Could you check a few things on this model? Use its own coordinates, in mm. Give positions to 0.01 mm unless a question says otherwise; leave off trailing zeros. Order: outer loops, then holes, each group sorted by start corner. A loop starts at its lowest first (then second) coordinate and runs counter-clockwise, first axis right, second up. Notation, with made-up numbers: (-12.5, 68) - (32.5, 68) arc R5 ccw to (32.5, 76) - close; hole circle Ø11 at (4, 82.5). An arc over 180 degrees is marked (long way). Put each result on its own line as item: value.
from build123d import *

# Parameters (mm, degrees)
F2_R     = 5.25
F4_R     = 25.9807621135
F5_DEPTH = 2.5


# Not quite as in the source:
# - a pattern or mirror of a feature is missing from the dataset's text; its kind, count and spacing are read off the source's solid


with BuildPart() as f1:
    # F0 (on Front) → F1 (revolve)
    with BuildSketch(Plane.XZ):
        with BuildLine():
            Line((-15, 25.9807621135), (-15, 0))
            Line((-15, 0), (15, 0))
            Line((15, 0), (15, 25.9807621135))
            ThreePointArc((15, 25.9807621135), (0, 30), (-15, 25.9807621135))
        make_face()
    revolve(axis=Axis((0, 0, 0), (1, 0, 0)))

    # F2 (on Right) → F3 (revolve, cut)
    with BuildSketch(Plane.YZ):
        with Locations((0, -27.5)):
            Circle(F2_R)
    f3 = revolve(axis=Axis((0, 15, 0), (0, 1, 0)), mode=Mode.SUBTRACT)

    # F3_copies: F3 across plane
    add(f3.mirror(Plane(origin=(0, -1e-06, -1e-06), x_dir=(0, -0.7071084838, 0.7071050786), z_dir=(0, -0.7071050786, -0.7071084838))), mode=Mode.SUBTRACT)

    # F4 (on face) → F5 (join)
    with BuildSketch(Plane(origin=(-15, 0, 0), x_dir=(0, -1, 0), z_dir=(-1, 0, 0))):
        Circle(F4_R)
    extrude(amount=-F5_DEPTH)

    # F6: F1 across plane


with BuildPart() as f1_1:
    add(f1.part)
    add(f1.part.mirror(Plane.YZ))


solid = f1_1.part
1) Suppose I cut it at A-A, the plane y = 1. List the corners of the cut face in (x, z) for me, and give its area (3 significant figures).
Filled in:
outline: (-15, -25.96) - (-12.5, -25.96) - (-12.5, -18.52) arc R22.35 ccw to (12.5, -18.52) - (12.5, -25.96) - (15, -25.96) - (15, 25.96) - (12.5, 25.96) - (12.5, 18.52) arc R22.35 ccw to (-12.5, 18.52) - (-12.5, 25.96) - (-15, 25.96) - close
area: 1,320 mm^2
2) Suppose I cut it at D-D, the plane z = 6. List the corners of the cut face in (x, y) for me.
Filled in:
outline: (-15, -25.28) arc R29.39 ccw to (15, -25.28) - (15, 25.28) arc R29.39 ccw to (-15, 25.28) - close
3) If I drill on line 1 (Z direction, x = 7, y = -21.5); line 2 (Z direction, x = -9, y = -25.5); line 3 (Z direction, x = 5, y = -5.5), over which ranges is the centre line in solid material (lowest first)? Write a range as [from, to].
Filled in:
line 1: z = [-19.72, -1.91], [1.91, 19.72]
line 2: z = [-12.99, -5.23], [5.23, 12.99]
line 3: z = [-29.06, 29.06]
4) Suppose I cut it at B-B, the plane z = -21.5. State how many separate pieces and enclosed holes the cut face has, and give its area (3 significant figures).
Filled in:
separate pieces: 1
enclosed holes: 2
area: 1,060 mm^2
5) We'd pull the mould along Y, two halves only. Please class faces 1 (the flat face through (-15, 0, 0)), 2 (the flat face through (12.5, 0, 23)): pulls with the +Y half, pulls with the -Y half, needs draft (parallel to the pull), parting line crosses it, or undercut.
Filled in:
face 1: needs draft
face 2: undercut
6) I'm going to push flat-ended pins straight in: pin 1 (1 mm diameter, centred on x = 0.5, z = 17.5, fed in from +Y); pin 2 (1 mm diameter, centred on x = 9.5, y = 10, fed in from +Z); pin 3 (2 mm diameter, centred on x = 10.5, z = 4, fed in from +Y). Where does each tip first touch, or does it pass through?
Filled in:
pin 1: stops at y = 24.71
pin 2: stops at z = 26.89
pin 3: stops at y = 27.91
